The listing builds one solid part. Answer for the finished solid, in the listing's coordinates (mm). Give positions to 0.01 mm unless a question says otherwise; leave off trailing zeros. Write each loop counter-clockwise with the first axis right and the second up, starting at its lowest first coordinate (ties: lowest second). Pieces come first, ordered by that corner, then holes. Notation, with made-up numbers: M 89,-24 L 110,-24 A21 ccw 110,12 Z; hole C -27.75,79 d8. An arc over 180 degrees is marked long. Answer as a JSON object with one key per item and string values.
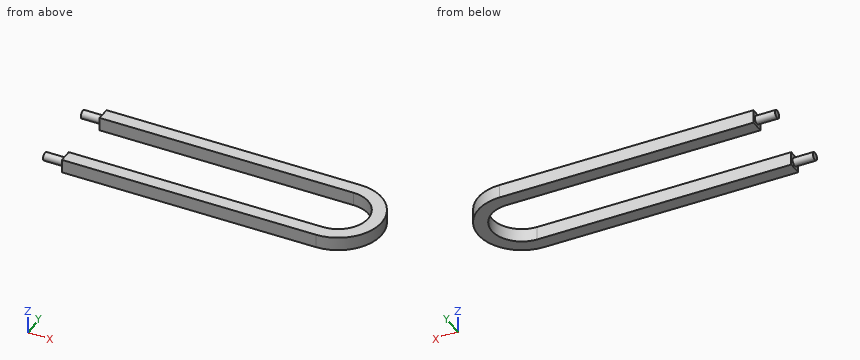
```python
from build123d import *

# Parameters (mm, degrees)
BOSS_EXTRUDE1_DEPTH = 10
SKETCH2_R           = 3
BOSS_EXTRUDE2_DEPTH = 15
SKETCH3_R           = 3
BOSS_EXTRUDE3_DEPTH = 15


with BuildPart() as part:
    # Sketch1 → Boss-Extrude1 (new body)
    with BuildSketch(Plane.XY):
        with BuildLine():
            Line((0, 0), (188.467924539, 0))
            ThreePointArc((188.467924539, 0), (220.672766762, -32.204842223), (188.467924539, -64.409684446))
            Line((188.467924539, -64.409684446), (0, -64.409684446))
            Line((0, -64.409684446), (0, -54.409684446))
            Line((0, -54.409684446), (188.467924539, -54.409684446))
            ThreePointArc((188.467924539, -54.409684446), (210.672766762, -32.204842223), (188.467924539, -10))
            Line((188.467924539, -10), (0, -10))
            Line((0, -10), (0, 0))
        make_face()
    extrude(amount=BOSS_EXTRUDE1_DEPTH)

    # Sketch2 → Boss-Extrude2 (add)
    with BuildSketch(Plane.ZY):
        with Locations(Location((5, -4.906979909, 0), (0, 0, 180))):
            Circle(SKETCH2_R)
    extrude(amount=BOSS_EXTRUDE2_DEPTH)

    # Sketch3 → Boss-Extrude3 (add)
    with BuildSketch(Plane.ZY):
        with Locations(Location((5, -59.409684446, 0), (0, 0, 180))):
            Circle(SKETCH3_R)
    extrude(amount=BOSS_EXTRUDE3_DEPTH)


solid = part.part
```
1. A cutting plane is placed at B-B, the plane z = 5. Give the vertices of the cut face in (x, y).
Verdict:
{"outline": "M -15,-62.41 L 0,-62.41 L 0,-64.41 L 188.47,-64.41 A32.2 ccw 188.47,0 L 0,0 L 0,-1.91 L -15,-1.91 L -15,-7.91 L 0,-7.91 L 0,-10 L 188.47,-10 A22.2 cw 188.47,-54.41 L 0,-54.41 L 0,-56.41 L -15,-56.41 Z"}
2. A cutting plane is placed at D-D, the plane y = -13. Give the vertices of the cut face in (x, z), plus the area to 3 significant figures.
Verdict:
{"outline": "M 199.61,0 L 214.32,0 L 214.32,10 L 199.61,10 Z", "area": "147 mm2"}
3. Consider line 1 along Y through (x, z) = (28, 6.5); line 2 along X through (y, z) = (-43, 4.25); line 3 along X through (y, z) = (-50.5, 1.5). Determine where each line is inside the solid, lowest interval first.
Verdict:
{"line 1": "y = -64.41 to -54.41, -10 to 0", "line 2": "x = 207.87 to 218.81", "line 3": "x = 201.05 to 214.97"}
4. A cutting plane is placed at C-C, the plane y = -28. Give the vertices of the cut face in (x, z).
Verdict:
{"outline": "M 210.27,0 L 220.4,0 L 220.4,10 L 210.27,10 Z"}
5. A cutting plane is placed at A-A, the plane x = 129.5. Give the vertices of the cut face in (y, z).
Verdict:
{"outline": "M -64.41,0 L -54.41,0 L -54.41,10 L -64.41,10 Z; M -10,0 L 0,0 L 0,10 L -10,10 Z"}
6. Flat-ended cylindrical pins translate along their axes: pin 1 (1.5 mm diameter, centred on y = -30.5, z = 6, fed in from -X); pin 2 (1 mm diameter, centred on y = -32, z = 7, fed in from -X). Find the tip coordinate at first contact, or state that the pin passes through.
Verdict:
{"pin 1": "stops at x = 210.54", "pin 2": "stops at x = 210.66"}
